Check sheet for the modelled part. Datum: model origin and axes. Units: mm. A direction names the side the tool comes from. Give positions to 0.01 mm unless a question says otherwise; leave off trailing zeros. Order: outer loops, then holes, each group sorted by start corner. A loop starts at its lowest first (then second) coordinate and runs counter-clockwise, first axis right, second up.
from build123d import *

# Parameters (mm, degrees)
F0_W     = 40
F0_H     = 40
F1_DEPTH = 40
F2_R     = 19.99999
F3_W     = 40
F3_H     = 40
F4_DEPTH = 25
F6_DEPTH = 25
F7_DEPTH = 50


# Not quite as in the source:
# - a fillet or chamfer is up to 0.001 mm smaller than in the source, because OpenCascade refuses the exact size


with BuildPart() as f1:
    # F0 (on Front) → F1 (new body)
    with BuildSketch(Plane.XZ):
        Rectangle(F0_W, F0_H)
    extrude(amount=F1_DEPTH)

    # F2 (radius 20 in the source; OpenCascade refuses exactly that, so slightly less here)
    f2_edges = [f1.edges().sort_by_distance(p)[0] for p in [
        (20, -20, 20),
        (-20, -20, 20),
        (0, 0, 20),
        (0, -40, 20),
        (0, -40, -20),
        (20, -40, 0),
        (-20, -40, 0),
        (20, -20, -20),
        (20, 0, 0),
        (0, 0, -20),
        (-20, 0, 0),
        (-20, -20, -20),
    ]]
    fillet(f2_edges, radius=F2_R)

    # F3 (on Top) → F4 (join)
    with BuildSketch(Plane.XY):
        with Locations((0, -20)):
            Rectangle(F3_W, F3_H)
    extrude(amount=F4_DEPTH)

    # F5 (on Right) → F6 (join)
    with BuildSketch(Plane.YZ):
        Polygon((-25, 0), (-20, 0), (-15, 0), (-15, 7.5), (0, 7.5), (0, 17.5), (-15, 17.5), (-15, 25), (-25, 25), (-25, 17.5), (-40, 17.5), (-40, 7.5), (-25, 7.5), align=None)
    extrude(amount=F6_DEPTH)

    # F7 (add): a face of the model
    f7_faces = [f1.faces().sort_by_distance(p)[0] for p in [
        (25, -20, 12.5),
    ]]
    extrude(f7_faces, amount=-F7_DEPTH)


solid = f1.part
1) Depth check by flat-ended pin: pin 1 Ø2.5 at (x, z) = (23, 22) entering from -Y; pin 2 Ø5.5 at (x, y) = (-23.5, -32) entering from +Z; pin 3 Ø3 at (x, y) = (17.5, -24) entering from -Z. Enter the tip coordinate at first touch or a pass-through.
Recorded:
pin 1: stops at y = -25
pin 2: stops at z = 17.5
pin 3: stops at z = -11.37
2) Material ranges on L1, parallel to X at y = -13, z = 22; L2, parallel to Z at x = 16, y = -4; L3, parallel to Z at x = -16.5, y = -16, recorded low to high.
Recorded:
L1: x = -20 to 20
L2: z = 0 to 25
L3: z = -10.57 to 25
3) Section check A-A, the plane z = 1.5. Record the cut outline in (x, y), then the cut area to 3 significant figures.
Recorded:
outline: (-25, -25) - (-20, -25) - (-20, -40) - (20, -40) - (20, -25) - (25, -25) - (25, -15) - (20, -15) - (20, 0) - (-20, 0) - (-20, -15) - (-25, -15) - close
area: 1,700 mm2
4) Set-up check for faces 1 (the face through (22, -25, 21)), 2 (the face through (-22, -25, 21)), 3 (the face through (22, -25, 4)), 4 (the face through (-22, -8, 7.5)): record each of +Z, -Z, +X, -X, +Y, -Y from which the full face is reachable in a straight line by a thin tool's end or side.
Recorded:
face 1: +Z, +X, -Y
face 2: +Z, -X, -Y
face 3: -Z, +X, -Y
face 4: -Z, -X, +Y
